The figure shows three views and two pictorial views of one solid part (mm, origin at its lowest corner). Answer the questions. A direction names the side the tool comes from. Round coordinates to 2 decimals unless told otherwise and drop trailing zeros. Order: outer loops, then holes, each group sorted by start corner. A loop starts at its lowest first (then second) coordinate and runs counter-clockwise, first axis right, second up. Notation, with made-up numbers: (-20.5, 34.5) -> (-14.5, 34.5) arc R23 ccw to (-14.5, 63.5) -> close; hole circle Ø5 at (55, 4). An arc over 180 degrees is marked (long way). Return JSON: item names as keys, results as strings. Group by question number.
(1) Consider line 1 (X direction, y = 3.9, z = 29); line 2 (Y direction, x = 43.25, z = 34.6); line 3 (X direction, y = 44, z = 36.7). Determine where each line is inside the solid, lowest interval first. Write a range as [from, to].
(2) The part is cut by section C-C (z = 29). Determine the outline of the cut face in (x, y), plus the area to 3 significant figures.
(3) The part is cut by section D-D (y = 44). Determine the outline of the cut face in (x, z).
(4) Which of the six approach directions +Z, -Z, +X, -X, +Y, -Y give full straight-line access (tool end or side, diameter ignored) to the marked faces 1, 2 and 3?
(5) Each of these flat-tipped pins is pushed along its axis until it touches: pin 1 (8 mm diameter, centred on x = 18, z = 27, fed in from +Y); pin 2 (2 mm diameter, centred on x = 3.25, y = 44, fed in from -Z); pin 3 (0.6 mm diameter, centred on x = 23, z = 35, fed in from +Y); pin 4 (1.5 mm diameter, centred on x = 22.5, z = 15, fed in from +Y). Where does it stop, or does it pass through?
(6) The part is cut by section B-B (y = 29). Determine the outline of the cut face in (x, z), plus the area to 4 significant figures.
(7) The part is cut by section A-A (x = 3.25). Determine the outline of the cut face in (y, z), plus the area to 3 significant figures.
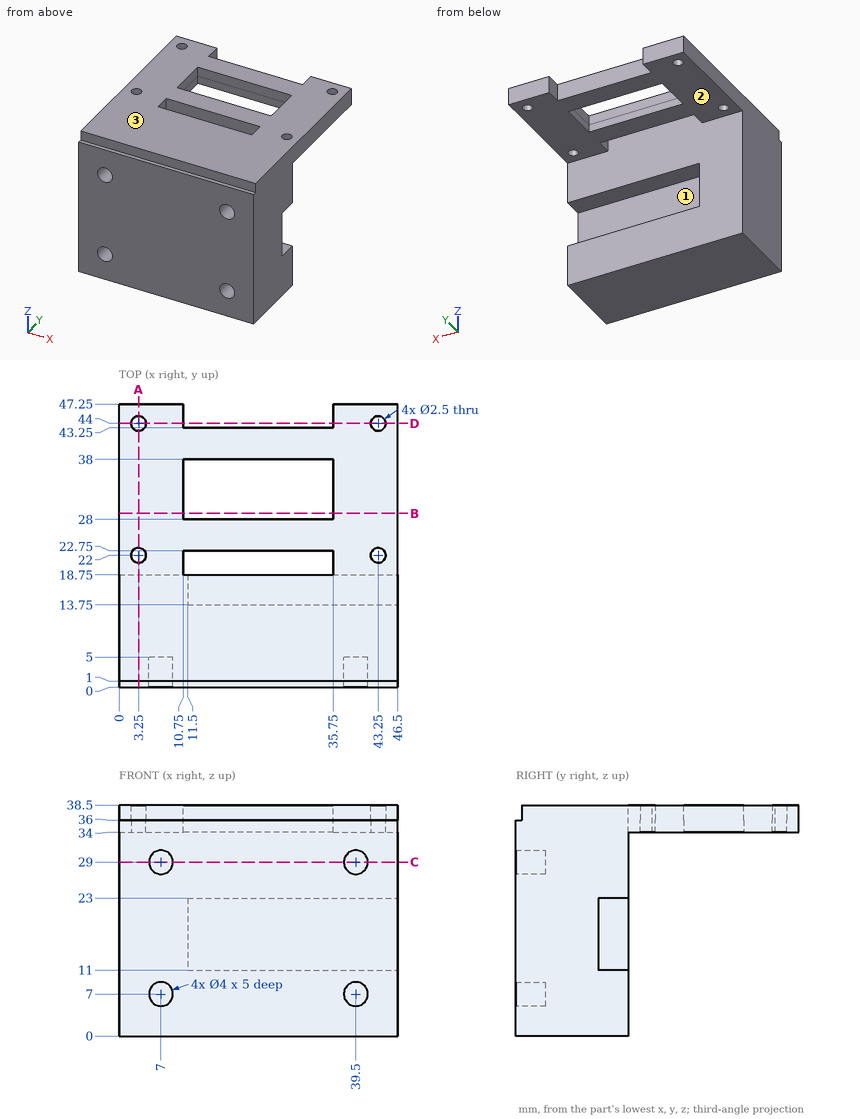
Answer below:
{
 "1": {"line 1": "x = [0, 5], [9, 37.5], [41.5, 46.5]", "line 2": "y = [0, 20.75], [23.25, 42.75], [45.25, 47.25]", "line 3": "x = [0, 2], [4.5, 10.75], [35.75, 42], [44.5, 46.5]"},
 "2": {"outline": "(0, 0) -> (5, 0) -> (5, 5) -> (9, 5) -> (9, 0) -> (37.5, 0) -> (37.5, 5) -> (41.5, 5) -> (41.5, 0) -> (46.5, 0) -> (46.5, 18.75) -> (0, 18.75) -> close", "area": "832 mm²"},
 "3": {"outline": "(0, 34) -> (2, 34) -> (2, 38.5) -> (0, 38.5) -> close; (4.5, 34) -> (10.75, 34) -> (10.75, 38.5) -> (4.5, 38.5) -> close; (35.75, 34) -> (42, 34) -> (42, 38.5) -> (35.75, 38.5) -> close; (44.5, 34) -> (46.5, 34) -> (46.5, 38.5) -> (44.5, 38.5) -> close"},
 "4": {"face 1": "+X, +Y", "face 2": "-Z, +X, -X, +Y", "face 3": "+Z, +X, -X, +Y, -Y"},
 "5": {"pin 1": "stops at y = 18.75", "pin 2": "passes through", "pin 3": "stops at y = 43.25", "pin 4": "stops at y = 13.75"},
 "6": {"outline": "(0, 34) -> (10.75, 34) -> (10.75, 38.5) -> (0, 38.5) -> close; (35.75, 34) -> (46.5, 34) -> (46.5, 38.5) -> (35.75, 38.5) -> close", "area": "96.75 mm²"},
 "7": {"outline": "(0, 0) -> (18.75, 0) -> (18.75, 34) -> (20.75, 34) -> (20.75, 38.5) -> (1, 38.5) -> (1, 36) -> (0, 36) -> close; (23.25, 34) -> (42.75, 34) -> (42.75, 38.5) -> (23.25, 38.5) -> close; (45.25, 34) -> (47.25, 34) -> (47.25, 38.5) -> (45.25, 38.5) -> close", "area": "825 mm²"}
}
